Geometry check sheet. Reference: the model listing, model coordinates, mm. A direction names the side the tool comes from. Round coordinates to 2 decimals unless told otherwise and drop trailing zeros. Order: outer loops, then holes, each group sorted by start corner. A loop starts at its lowest first (then second) coordinate and runs counter-clockwise, first axis right, second up. Notation, with made-up numbers: (-30, -9) -> (29, -9) arc R26 cw to (29, 26) -> close; hole circle Ø5 at (12.25, 77). An arc over 180 degrees is marked (long way). Answer as a JSON object with one key per item and string values. Group by question number.
Autodesk Fusion 360 part; units mm, degrees
sketch "Sketch1" plane through (0, 0, 0) normal (0, 0, 1) x (1, 0, 0)
  line L0 (160, -90) -> (-160, -90)
  line L1 (-160, -90) -> (-160, 90)
  line L2 (-160, 90) -> (160, 90)
  line L3 (160, 90) -> (160, -90)
  line L4 (160, -90) -> (-160, 90) construction
  line L5 (-160, -90) -> (160, 90) construction
  line L6 (170, 85.5) -> (-180, 85.5) construction
  line L7 (-180, -85.5) -> (170, -85.5) construction
  line L8 (-155.5, 90) -> (-155.5, -90)
  line L9 (-160, 90) -> (-135, 90)
  line L10 (-135, 90) -> (-135, 85.5)
  line L11 (-135, 85.5) -> (-160, 85.5)
  line L12 (-160, 85.5) -> (-160, 90)
  line L13 (-160, -90) -> (-135, -90)
  line L14 (-135, -90) -> (-135, -85.5)
  line L15 (-135, -85.5) -> (-160, -85.5)
  line L16 (-160, -85.5) -> (-160, -90)
  line L17 (-110, -90) -> (-10, -90)
  line L18 (-10, -90) -> (-10, -85.5)
  line L19 (-10, -85.5) -> (-110, -85.5)
  line L20 (-110, -85.5) -> (-110, -90)
  line L21 (-10, -90) -> (15, -90)
  line L22 (15, -90) -> (15, -85.5)
  line L23 (15, -85.5) -> (-10, -85.5)
  line L24 (-10, -85.5) -> (-10, -90)
  line L25 (15, -90) -> (115, -90)
  line L26 (115, -85.5) -> (15, -85.5)
  line L27 (15, -85.5) -> (15, -90)
  line L28 (115, -90) -> (140, -90)
  line L29 (140, -85.5) -> (115, -85.5)
  line L30 (-135, 85.5) -> (-110, 85.5)
  line L31 (-110, 85.5) -> (-110, 90)
  line L32 (-110, 90) -> (-135, 90)
  line L33 (-135, 90) -> (-135, 85.5)
  line L34 (-110, 85.5) -> (-10, 85.5)
  line L35 (-10, 85.5) -> (-10, 90)
  line L36 (-10, 90) -> (-110, 90)
  line L37 (-110, 90) -> (-110, 85.5)
  line L38 (-10, 85.5) -> (15, 85.5)
  line L39 (15, 85.5) -> (15, 90)
  line L40 (15, 90) -> (-10, 90)
  line L41 (-10, 90) -> (-10, 85.5)
  line L42 (15, 85.5) -> (115, 85.5)
  line L43 (115, 90) -> (15, 90)
  line L44 (15, 90) -> (15, 85.5)
  line L45 (115, 85.5) -> (140, 85.5)
  line L46 (140, 90) -> (115, 90)
  line L47 (140, 85.5) -> (160, 85.5)
  line L48 (160, 85.5) -> (160, 90)
  line L49 (160, 90) -> (140, 90)
  line L50 (140, -90) -> (160, -90)
  line L51 (160, -90) -> (160, -85.5)
  line L52 (160, -85.5) -> (140, -85.5)
  line L53 (-160, 55) -> (-155.5, 55)
  line L54 (-155.5, 55) -> (-155.5, 35)
  line L55 (-155.5, 35) -> (-160, 35)
  line L56 (-160, 35) -> (-160, 55)
  line L57 (-160, -35) -> (-155.5, -35)
  line L58 (-155.5, -35) -> (-155.5, -55)
  line L59 (-155.5, -55) -> (-160, -55)
  line L60 (-160, -55) -> (-160, -35)
  line L61 (30, 90) -> (30, -90)
  line L62 (30, -75.5) -> (25, -75.5)
  line L63 (25, -75.5) -> (25, -21.5)
  line L64 (25, -21.5) -> (30, -21.5)
  line L65 (30, -21.5) -> (30, -75.5)
  point P0 (-15, -14)
  dimension "d1" = 320
  dimension "d2" = 180
  dimension "d3" = 4.5
  dimension "d4" = 4.5
  dimension "d5" = 4.5
  dimension "d6" = 25
  dimension "d7" = 25
  dimension "d8" = 100
  dimension "d9" = 25
  dimension "d10" = 25
  dimension "d13" = 25
  dimension "d14" = 100
  dimension "d15" = 25
  dimension "d18" = 20
  dimension "d19" = 20
  dimension "d20" = 35
  dimension "d21" = 35
  dimension "d46" = 15
  dimension "d55" = 5
  dimension "d56" = 54
  dimension "d58" = 10
extrude "Extrude1" add sketch "Sketch1" along normal blind 4.5 contours L0 L18 L21 L22 L23 L24 L27 | L0 L8 L11 L14 L15 L19 L20 L23 L26 L30 L34 L38 L42 L54 L58 L61 L62 L63 L64 | L2 L35 L38 L39 L40 L41 L44 | L2 L10 L30 L31 L32 L33 L37 | L1 L8 L57 L58 L59 L60 | L1 L8 L53 L54 L55 L56
move_face "OffsetFaces1" offset -0.1 4 faces at (15, -88.5, 1.5) (-110, -87, 1.5) (-110, 87, 1.5) (15, 87, 1.5)
move_face "OffsetFaces2" offset -0.1 4 faces at (-10, -88.5, 1.5) (-135, -88.5, 1.5) (-10, 87, 1.5) (-135, 88.5, 1.5)
move_face "OffsetFaces3" offset -0.1 2 faces at (-158.5, -35, 1.5) (-158.5, 55, 1.5)
move_face "OffsetFaces4" offset -0.1 2 faces at (-157, -55, 1.5) (-157, 35, 1.5)
fillet "Fillet1" radius 2 2 edges at (25, -75.5, 2.25) (25, -21.5, 2.25)
Item 1: Mould release check, pull along X, two halves, no side actions. Record for faces 4 (the flat face through (-155.5, -70, 2)), 5 (the flat face through (-66, 1, 0)), 6 (the flat face through (30, -80, 2)), 7 (the flat face through (-61, 85.5, 2)): pulls with the +X half, pulls with the -X half, needs draft (parallel to the pull), parting line crosses it, or undercut.
Item 2: Sectioned sample at B-B, the plane y = -66.5. Enter the section's corners in (x, z).
Item 3: Set-up check for faces 1 (the flat face through (25, -49, 2)), 2 (the flat face through (14.9, -88, 2)), 3 (the flat face through (-158, 54.9, 2)): record each of +Z, -Z, +X, -X, +Y, -Y from which the full face is reachable in a straight line by a thin tool's end or side.
Item 4: Sectioned sample at C-C, the plane x = -67.5. Enter the section's corners in (y, z).
Item 5: Depth check by flat-ended pin: pin 1 Ø2 at (x, z) = (-67, 2.5) entering from +Y; pin 2 Ø2 at (x, z) = (-142.5, 2.5) entering from -Y; pin 3 Ø2 at (y, z) = (-87.5, 3) entering from +X. Enter the tip coordinate at first touch or a pass-through.
Item 6: Thickness scan on L1, parallel to Y at x = -19, z = 0.4; L2, parallel to X at y = 28, z = 0.9; L3, parallel to X at y = -33.5, z = 3.15. Record the ranges inside material, lowest first.
Result:
{
 "1": {"face 4": "pulls with the -X half", "face 5": "needs draft", "face 6": "pulls with the +X half", "face 7": "undercut"},
 "2": {"outline": "(-155.5, 0) -> (25, 0) -> (25, 4.5) -> (-155.5, 4.5) -> close"},
 "3": {"face 1": "+Z, -Z, +X", "face 2": "+Z, -Z, +X, -Y", "face 3": "+Z, -Z, -X, +Y"},
 "4": {"outline": "(-85.5, 0) -> (85.5, 0) -> (85.5, 4.5) -> (-85.5, 4.5) -> close"},
 "5": {"pin 1": "stops at y = 85.5", "pin 2": "stops at y = -85.5", "pin 3": "stops at x = 14.9"},
 "6": {"L1": "y = -85.5 to 85.5", "L2": "x = -155.5 to 30", "L3": "x = -155.5 to 25"}
}
